Check sheet for the modelled part. Datum: model origin and axes. Units: mm. Face numbers are marked on the shaded views. Give positions to 0.01 mm unless a question says otherwise; leave off trailing zeros. Write each loop counter-clockwise with the first axis right and the second up, starting at its lowest first coordinate (ties: lowest second). Pieces come first, ordered by that corner, then holes. Notation, with made-up numbers: M -21.75,39 L 13.25,39 A19 cw 13.25,53 Z; hole C 56.25,9.25 d3. An arc over 180 degrees is marked long. Write item = value, one per line. Start each with the question number.
1) Cross-section at C-C, the plane z = -54. Record the cut outline in (x, y).
2) Cross-section at A-A, the plane y = 0. Record the cut outline in (x, z).
3) Mould release check, pull along Z, two halves, no side actions. Record for the marked faces 1, 2 and 3: released by +Z, released by -Z, zero draft, split by the parting line, or undercut.
4) Cross-section at B-B, the plane x = 0. Record the cut outline in (y, z).
5) Scan lines: line 1 along Z through (x, y) = (4.5, 7.25); line 2 along Z through (x, y) = (0, -6.75); line 3 along X through (y, z) = (0.25, 31.5). Record each from-to range of solid material in increasing order. Write a range as [from, to].
6) Go/stop test with flat-tipped pins: pin 1 (5 mm diameter, centred on y = -5.5, z = -96.5, fed in from -X); pin 2 (3 mm diameter, centred on x = -5.5, z = -84.5, fed in from -Y); pin 3 (6 mm diameter, centred on x = -1, z = 65.5, fed in from -Y). Record where each tip stops, or that it passes through.
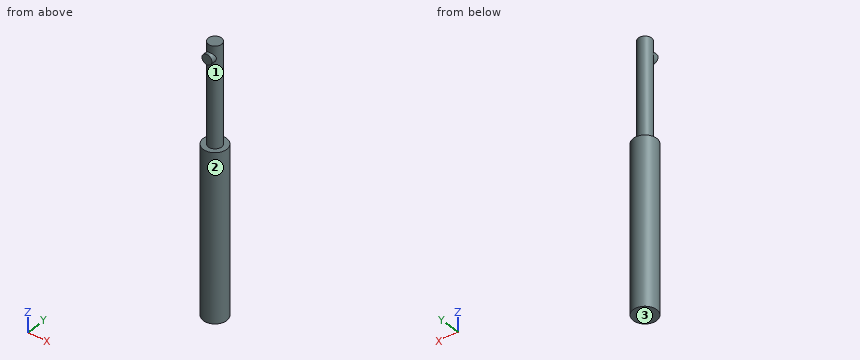
```python
from build123d import *

# Parameters (mm, degrees)
F0_R     = 8.89
F1_DEPTH = 127
F2_R     = 5.08
F3_DEPTH = 76.2
F4_R     = 3.81
F5_DEPTH = 7.62


with BuildPart() as f1:
    # F0 (on Top) → F1 (new body)
    with BuildSketch(Plane.XY):
        Circle(F0_R)
    extrude(amount=-F1_DEPTH)

    # F2 (on Top) → F3 (join)
    with BuildSketch(Plane.XY):
        Circle(F2_R)
    extrude(amount=F3_DEPTH)

    # F4 (on Front) → F5 (join)
    with BuildSketch(Plane.XZ):
        with Locations((0, 66.903524)):
            Circle(F4_R)
    extrude(amount=F5_DEPTH)


solid = f1.part
```
Reply:
q1.outline = C 0,0 d17.78
q2.outline = M -8.89,-127 L 8.89,-127 L 8.89,0 L 5.08,0 L 5.08,76.2 L -5.08,76.2 L -5.08,0 L -8.89,0 Z
q3.face_1 = undercut
q3.face_2 = zero draft
q3.face_3 = released by -Z
q4.outline = M -8.89,-127 L 8.89,-127 L 8.89,0 L 5.08,0 L 5.08,76.2 L -5.08,76.2 L -5.08,70.71 L -7.62,70.71 L -7.62,63.09 L -5.08,63.09 L -5.08,0 L -8.89,0 Z
q5.line_1 = [-127, 0]
q5.line_2 = [-127, 0], [63.09, 70.71]
q5.line_3 = [-5.07, 5.07]
q6.pin_1 = -8.37
q6.pin_2 = -7.94
q6.pin_3 = -7.62
